Work out the finished part from the listing and answer in its coordinate system (mm). Face numbers are marked on the shaded views. A direction names the side the tool comes from. Give positions to 0.01 mm unless a question says otherwise; leave off trailing zeros. Order: outer loops, then holes, each group sorted by start corner. A loop starts at its lowest first (then second) coordinate and runs counter-clockwise, first axis right, second up. Notation, with made-up numbers: M 83,5.25 L 121,5.25 A24 cw 121,15.25 Z; hole C 70,61 d8. An arc over 180 degrees is marked long. One line per item, written item: value.
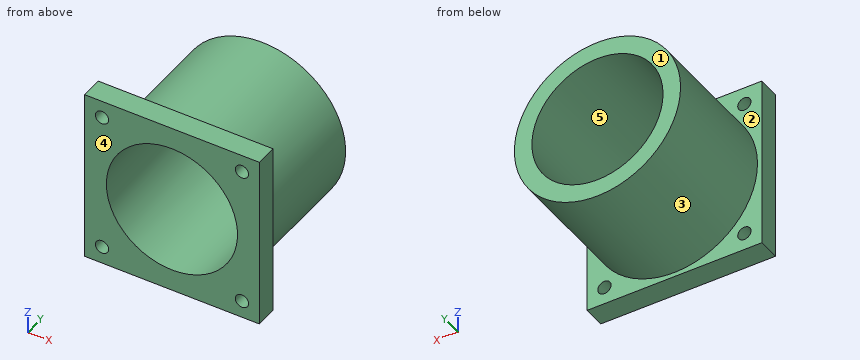
Autodesk Inventor part; units mm, degrees
ref_plane "YZ Plane" through (0, 0, 0) normal (1, 0, 0) x (0, 1, 0)
ref_plane "XZ Plane" through (0, 0, 0) normal (0, 1, 0) x (-1, 0, 0)
ref_plane "XY Plane" through (0, 0, 0) normal (0, 0, 1) x (1, 0, 0)
sketch "Sketch1" plane through (0, 0, 0) normal (0, 1, 0) x (-1, 0, 0)
  circle A0 centre (0, 0) radius 19.05
  circle A1 centre (0, 0) radius 24.13
  line L0 (25.4, 25.4) -> (-25.4, 25.4)
  line L1 (-25.4, 25.4) -> (-25.4, -25.4)
  line L2 (-25.4, -25.4) -> (25.4, -25.4)
  line L3 (25.4, -25.4) -> (25.4, 25.4)
  line L4 (-25.4, -25.4) -> (-12.1092, -25.4) construction
  circle A2 centre (-20.32, -20.32) radius 1.9304
  circle A3 centre (-20.32, 20.32) radius 1.9304
  circle A4 centre (20.32, -20.32) radius 1.9304
  circle A5 centre (20.32, 20.32) radius 1.9304
  dimension "d10" = 50.8
  dimension "d11" = 50.8
  dimension "d20" = 3.8608
  dimension "d25" = 3.8608
  dimension "d26" = 3.8608
  dimension "d27" = 3.8608
extrude "Extrusion1" add sketch "Sketch1" along normal blind 42.164 contours A1
extrude "Extrusion3" add sketch "Sketch1" along normal blind 6.35 contours A1 | L3 L2 L1 L0 | A2 | A3 | A4 | A5
extrude "Extrusion5" cut sketch "Sketch1" along normal blind 6.35 contours A2 | A3 | A4 | A5
properties part number "Cylinders"
(1) Given P1, Ø4.5, axis at x = 20.32, z = -20.32, coming from the +Y side; P2, Ø5, axis at x = 18, z = -2.5, coming from the -Y side; P3, Ø2, axis at y = 37, z = 10, coming from the +X side; P4, Ø4, axis at y = 13, z = -4.5, coming from the +X side, each flat-ended and moving along its own axis, determine where each tip first touches the part or whether it passes through.
Findings:
P1: stops at y = 6.35
P2: stops at y = 0
P3: stops at x = 22.39
P4: stops at x = 24
(2) Which of the six approach directions +Z, -Z, +X, -X, +Y, -Y give full straight-line access (tool end or side, diameter ignored) to the marked faces 1 and 2?
Findings:
face 1: +Z, -Z, +X, -X, +Y
face 2: +Y
(3) Section B-B, the plane x = 0 is taken. Give the vertices of the cut face in (y, z).
Findings:
outline: M 0,-25.4 L 6.35,-25.4 L 6.35,-24.13 L 42.16,-24.13 L 42.16,-19.05 L 0,-19.05 Z; M 0,19.05 L 42.16,19.05 L 42.16,24.13 L 6.35,24.13 L 6.35,25.4 L 0,25.4 Z
(4) Section C-C, the plane y = 5.5 is taken. Give the vertices of the cut face in (x, z).
Findings:
outline: M -25.4,-25.4 L 25.4,-25.4 L 25.4,25.4 L -25.4,25.4 Z; hole C -20.32,-20.32 d3.86; hole C -20.32,20.32 d3.86; hole C 0,0 d38.1; hole C 20.32,-20.32 d3.86; hole C 20.32,20.32 d3.86
(5) Section D-D, the plane z = -21 is taken. Give the vertices of the cut face in (x, y).
Findings:
outline: M -25.4,0 L -22.13,0 L -22.13,6.35 L -25.4,6.35 Z; M -18.51,0 L 18.51,0 L 18.51,6.35 L 11.89,6.35 L 11.89,42.16 L -11.89,42.16 L -11.89,6.35 L -18.51,6.35 Z; M 22.13,0 L 25.4,0 L 25.4,6.35 L 22.13,6.35 Z
(6) Section A-A, the plane z = 0 is taken. Give the vertices of the cut face in (x, y), then the cut area to 3 significant figures.
Findings:
outline: M -25.4,0 L -19.05,0 L -19.05,42.16 L -24.13,42.16 L -24.13,6.35 L -25.4,6.35 Z; M 19.05,0 L 25.4,0 L 25.4,6.35 L 24.13,6.35 L 24.13,42.16 L 19.05,42.16 Z
area: 445 mm^2
(7) Find the intervals of material crossed by probe 1 along Y at (x, z) = (-17, -19); probe 2 along X at (y, z) = (13.5, -10.5); probe 3 along X at (y, z) = (8.5, 15), in increasing order. Write a range as from..to.
Findings:
probe 1: y = 0..6.35
probe 2: x = -21.73..-15.9, 15.9..21.73
probe 3: x = -18.9..-11.74, 11.74..18.9
(8) Determine the mould class of the marked faces 3, 4 and 5 for opening direction X: pulls with the +X half, pulls with the -X half, needs draft (parallel to the pull), parting line crosses it, or undercut.
Findings:
face 3: parting line crosses it
face 4: needs draft
face 5: undercut
